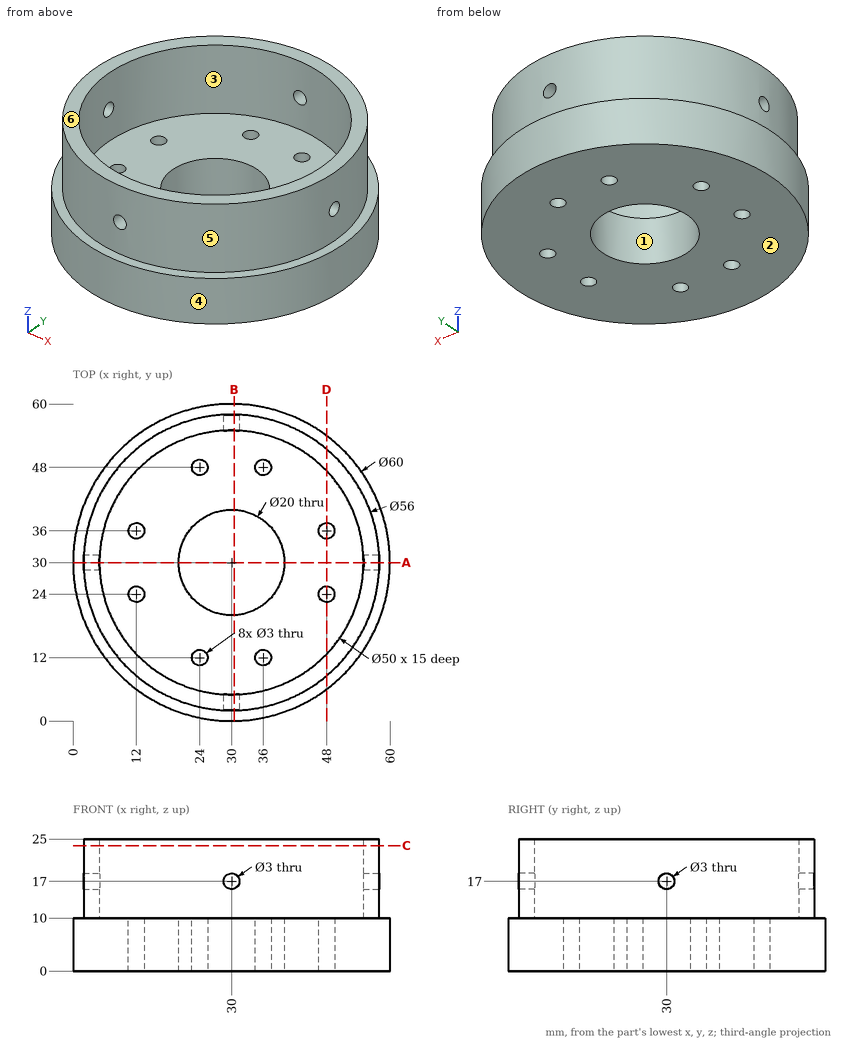
Here's the drawing with two shaded views (mm, measured from the low corner). I have some questions. A direction names the side the tool comes from. Coordinates: 2 decimals unless noted, no trailing zeros. Loops run counter-clockwise (first coordinate to the right, second up) from the corner with the lowest first, then second, coordinate; pieces in that order, holes last. Notation, with made-up numbers: (32, 8.5) -> (36, 8.5) arc R8 cw to (36, 21.5) -> close; hole circle Ø8 at (39, 28). An arc over 180 degrees is marked (long way). Answer as a JSON object with one key per item and string values.
1) Imagine slicing it at A-A (y = 30). Please give me the cut outline in (x, z), then the cut area to 3 significant figures.
Results:
{"outline": "(0, 0) -> (20, 0) -> (20, 10) -> (5, 10) -> (5, 15.5) -> (2, 15.5) -> (2, 10) -> (0, 10) -> close; (2, 18.5) -> (5, 18.5) -> (5, 25) -> (2, 25) -> close; (40, 0) -> (60, 0) -> (60, 10) -> (58, 10) -> (58, 15.5) -> (55, 15.5) -> (55, 10) -> (40, 10) -> close; (55, 18.5) -> (58, 18.5) -> (58, 25) -> (55, 25) -> close", "area": "472 mm^2"}
2) Imagine slicing it at B-B (x = 30.5). Please give me the cut outline in (y, z) (1 decimal).
Results:
{"outline": "(0, 0) -> (20, 0) -> (20, 10) -> (5, 10) -> (5, 15.6) -> (2, 15.6) -> (2, 10) -> (0, 10) -> close; (2, 18.4) -> (5, 18.4) -> (5, 25) -> (2, 25) -> close; (40, 0) -> (60, 0) -> (60, 10) -> (58, 10) -> (58, 15.6) -> (55, 15.6) -> (55, 10) -> (40, 10) -> close; (55, 18.4) -> (58, 18.4) -> (58, 25) -> (55, 25) -> close"}
3) For the marked faces 5 and 6, which set-ups out of +Z, -Z, +X, -X, +Y, -Y let a thin tool reach every point of the face, with its end or its side?
Results:
{"face 5": "+Z", "face 6": "+Z, +X, -X, +Y, -Y"}
4) For P1, Ø3.5, axis at x = 36, y = 48, coming from the +Z side; P2, Ø6, axis at x = 9, z = 13.5, coming from the +Y side; P3, Ø3, axis at x = 11.5, z = 4, coming from the -Y side, each with a flat end and sliding along its axis, tell me the tip position at first contact or that it passes through.
Results:
{"P1": "stops at z = 10", "P2": "stops at y = 51.45", "P3": "stops at y = 5.28"}
5) Thinking about a two-plate mould opening in Y: for the marked faces 1, 2, 3 and 4, which applies, pulls with the +Y half, pulls with the -Y half, needs draft (parallel to the pull), parting line crosses it, or undercut?
Results:
{"face 1": "undercut", "face 2": "needs draft", "face 3": "undercut", "face 4": "parting line crosses it"}
6) Imagine slicing it at D-D (x = 48). Please give me the cut outline in (y, z), then the cut area to 3 significant figures.
Results:
{"outline": "(6, 0) -> (22.5, 0) -> (22.5, 10) -> (12.65, 10) -> (12.65, 25) -> (8.55, 25) -> (8.55, 10) -> (6, 10) -> close; (25.5, 0) -> (34.5, 0) -> (34.5, 10) -> (25.5, 10) -> close; (37.5, 0) -> (54, 0) -> (54, 10) -> (51.45, 10) -> (51.45, 25) -> (47.35, 25) -> (47.35, 10) -> (37.5, 10) -> close", "area": "543 mm^2"}
7) If I drill on line 1 (Y direction, x = 48, z = 7); line 2 (Y direction, x = 30, z = 6); line 3 (X direction, y = 33, z = 15.5), over which ranges is the centre line in solid material (lowest first)?
Results:
{"line 1": "y = 6 to 22.5, 25.5 to 34.5, 37.5 to 54", "line 2": "y = 0 to 20, 40 to 60", "line 3": "x = 2.16 to 5.18, 54.82 to 57.84"}
8) Imagine slicing it at C-C (z = 23.75). Please give me the cut outline in (x, y), then the cut area to 3 significant figures.
Results:
{"outline": "circle Ø56 at (30, 30); hole circle Ø50 at (30, 30)", "area": "500 mm^2"}
